For this review, take the finished solid that the model builds, in its own axes (mm). Face numbers are marked on the shaded views. A direction names the side the tool comes from. Round coordinates to 2 decimals unless told otherwise and drop trailing zeros. Order: outer loops, then holes, each group sorted by start corner. A loop starts at its lowest first (then second) coordinate and runs counter-clockwise, first axis right, second up. Notation, with made-up numbers: (78, -30) -> (90, -30) arc R26 cw to (90, 3) -> close; hole circle Ø2 at (65.25, -15). An arc over 180 degrees is marked (long way). Use a Markdown table: item, result. Add a question column.
1) Consider section D-D (x = -9.5). State the section outline as (y, z) points, plus the area to 3 significant figures.
2) Wall thickness on line 1 along Y through (x, z) = (-4.3, -3); line 2 along X through (y, z) = (3, 2); line 3 along Z through (x, y) = (1.5, 5.75): over which ranges is each line inside the solid? List them lowest first. Write a range as [from, to].
3) Consider section A-A (z = 3.25). State the section outline as (x, y) points.
4) Clearance check with flat-ended pins moving along their axes: P1, Ø2.5, axis at x = 12.5, y = 4, coming from the -Z side; P2, Ø1.5, axis at y = 2.5, z = 2, coming from the -X side; P3, Ø2, axis at x = 0.5, y = 3.5, coming from the -Z side; P4, Ø2.5, axis at y = 4, z = -3.5, coming from the +X side. State where each tip first meets the part, or that it passes through.
5) Consider section C-C (z = -5). State the section outline as (x, y) points.
6) Machinability: for the marked faces 1, 2, 3, 4 and 5, which of the approach directions +Z, -Z, +X, -X, +Y, -Y give a long, thin tool a straight path to every point of the face, cutting with its end or side? Answer none if there is none.
7) Draft analysis for pull direction Y (two halves, no side actions). For the marked faces 6, 7 and 8, state which applies: pulls with the +Y half, pulls with the -Y half, needs draft (parallel to the pull), parting line crosses it, or undercut.
8) Consider section B-B (y = 6). State the section outline as (x, z) points.
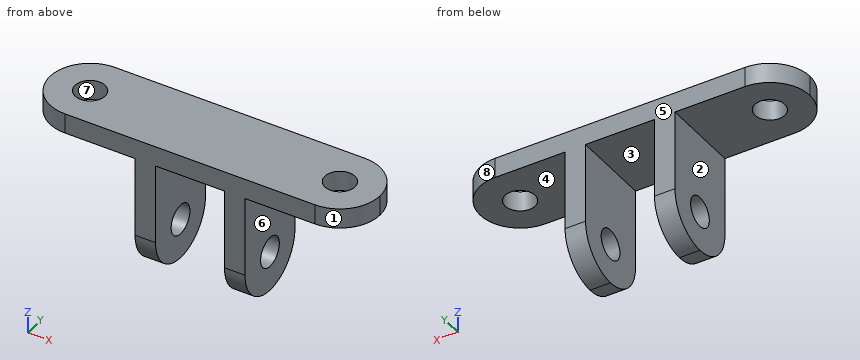
```python
from build123d import *

# Parameters (mm, degrees)
SKETCH_1_W          = 33
SKETCH_1_H          = 14
EXTRUDE_1_DEPTH     = 8
SKETCH_2_W          = 11
SKETCH_2_H          = 12
SKETCH_2_W_2        = 6.9
CUT_EXTRUDE_1_DEPTH = 20.627786426
FILLET_1_R          = 4
FILLET_2_R          = 4
SKETCH_3_R          = 1.5
CUT_EXTRUDE_2_DEPTH = 11
SKETCH_4_R          = 1.5
CUT_EXTRUDE_3_DEPTH = 24.07054399


with BuildPart() as part:
    # 草图1 → 凸台-拉伸1 (new body)
    with BuildSketch(Plane(origin=(0, 0, 0), x_dir=(1, 0, 0), z_dir=(0, 1, 0))):
        Rectangle(SKETCH_1_W, SKETCH_1_H)
    extrude(amount=EXTRUDE_1_DEPTH)

    # 草图2 → 切除-拉伸1 (cut, through all)
    with BuildSketch(Plane(origin=(0, 8, 0), x_dir=(1, 0, 0), z_dir=(0, 1, 0))):
        with Locations((-11, 1)):
            Rectangle(SKETCH_2_W, SKETCH_2_H)
        with Locations((11, 1)):
            Rectangle(SKETCH_2_W, SKETCH_2_H)
        with Locations((0, 1)):
            Rectangle(SKETCH_2_W_2, SKETCH_2_H)
    extrude(amount=-CUT_EXTRUDE_1_DEPTH, mode=Mode.SUBTRACT)

    # 圆角1
    fillet_1_edges = [part.edges().sort_by_distance(p)[0] for p in [
        (16.5, 0, 6),
        (16.5, 8, 6),
        (-16.5, 0, 6),
        (-16.5, 8, 6),
    ]]
    fillet(fillet_1_edges, radius=FILLET_1_R - 0.0001)  # a hair under: the kernel refuses the full size

    # 圆角2
    fillet_2_edges = [part.edges().sort_by_distance(p)[0] for p in [
        (-4.475, 8, -7),
        (-4.475, 0, -7),
        (4.475, 0, -7),
        (4.475, 8, -7),
    ]]
    fillet(fillet_2_edges, radius=FILLET_2_R - 0.0001)  # a hair under: the kernel refuses the full size

    # 草图3 → 切除-拉伸2 (cut)
    with BuildSketch(Plane(origin=(5.5, 0, 0), x_dir=(0, 0, -1), z_dir=(1, 0, 0))):
        with Locations((3, 4)):
            Circle(SKETCH_3_R)
    extrude(amount=-CUT_EXTRUDE_2_DEPTH, mode=Mode.SUBTRACT)

    # 草图4 → 切除-拉伸3 (cut, through all)
    with BuildSketch(Plane.XY.offset(7)):
        with Locations((12.5, 4)):
            Circle(SKETCH_4_R)
        with Locations((-12.5, 4)):
            Circle(SKETCH_4_R)
    extrude(amount=-CUT_EXTRUDE_3_DEPTH, mode=Mode.SUBTRACT)


solid = part.part
```
Results list:
| question | item | result |
|---|---|---|
| 1 | outline | (0, 5) -> (8, 5) -> (8, 7) -> (0, 7) -> close |
| 1 | area | 16.0 mm2 |
| 2 | line 1 | [0, 2.5], [5.5, 8] |
| 2 | line 2 | [-5.5, -3.45], [3.45, 5.5] |
| 2 | line 3 | [5, 7] |
| 3 | outline | (-5.5, 0) -> (-3.45, 0) -> (-3.45, 8) -> (-5.5, 8) -> close; (3.45, 0) -> (5.5, 0) -> (5.5, 8) -> (3.45, 8) -> close |
| 4 | P1 | through |
| 4 | P2 | x = -5.5 |
| 4 | P3 | z = 5 |
| 4 | P4 | x = 5.5 |
| 5 | outline | (-5.5, 0.54) -> (-3.45, 0.54) -> (-3.45, 7.46) -> (-5.5, 7.46) -> close; (3.45, 0.54) -> (5.5, 0.54) -> (5.5, 7.46) -> (3.45, 7.46) -> close |
| 6 | face 1 | +Z, -Z, +X, -Y |
| 6 | face 2 | -Z, -X, +Y, -Y |
| 6 | face 3 | -Z, +Y, -Y |
| 6 | face 4 | -Z, +X, +Y, -Y |
| 6 | face 5 | +Z, -Z, +X, -X, +Y |
| 7 | face 6 | needs draft |
| 7 | face 7 | undercut |
| 7 | face 8 | pulls with the +Y half |
| 8 | outline | (-15.96, 5) -> (-5.5, 5) -> (-5.5, -6.46) -> (-3.45, -6.46) -> (-3.45, 5) -> (3.45, 5) -> (3.45, -6.46) -> (5.5, -6.46) -> (5.5, 5) -> (15.96, 5) -> (15.96, 7) -> (-15.96, 7) -> close |
